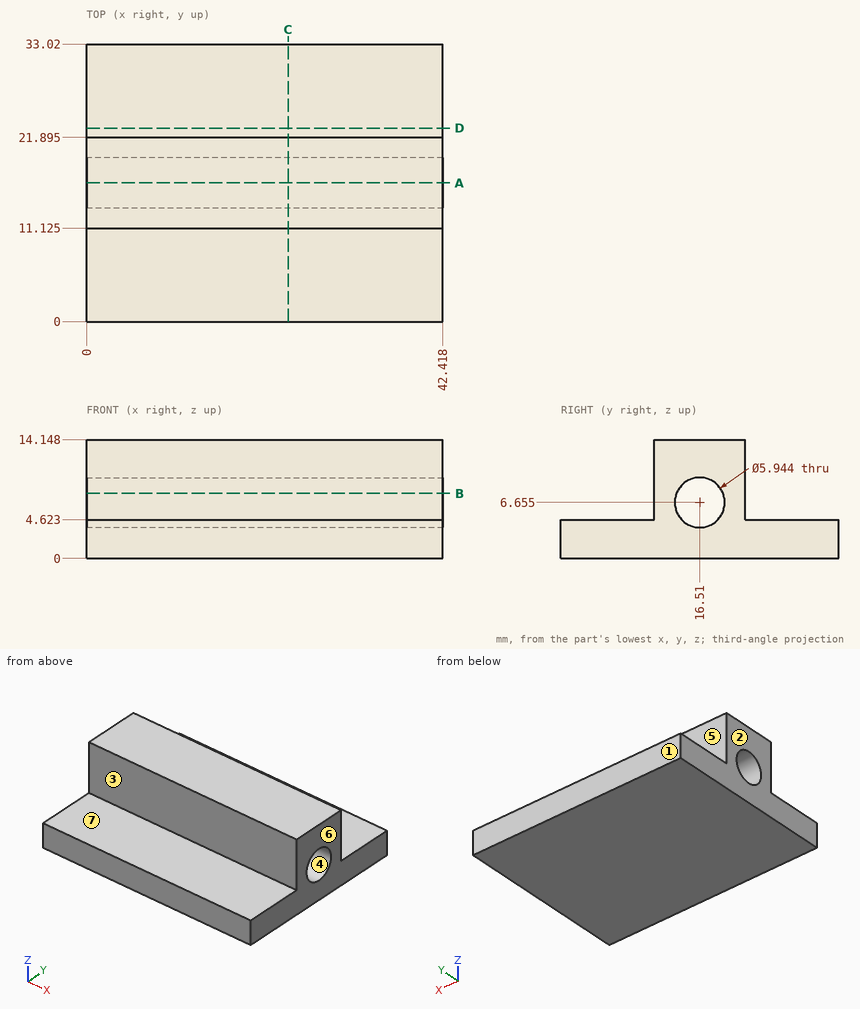
Verification items for this drawing (mm, ordinates from the low corner). A direction names the side the tool comes from. Coordinates: 2 decimals unless noted, no trailing zeros. Write each loop counter-clockwise with the first axis right and the second up, starting at its lowest first coordinate (ties: lowest second). Pieces come first, ordered by that corner, then holes. Notation, with made-up numbers: M 70,-5 L 126,-5 A29 ccw 126,17 Z; hole C 10,72 d6. An arc over 180 degrees is marked long. Answer as CSV lines item,"result".
Q1. Cross-section at D-D (y = 23). Record the boundary of the cut face in (x, z).
Check result:
outline,"M 0,0 L 42.42,0 L 42.42,4.62 L 0,4.62 Z"
Q2. Set-up check for the marked faces 5, 6 and 7: record each of +Z, -Z, +X, -X, +Y, -Y from which the full face is reachable in a straight line by a thin tool's end or side.
Check result:
face 5,"+Z, +X, -X, +Y"
face 6,"+Z, -Z, +X, +Y, -Y"
face 7,"+Z, +X, -X, -Y"
Q3. Material ranges on probe 1 along Y at (x, z) = (13.5, 11) (1 decimal); probe 2 along Z at (x, y) = (13, 16.51); probe 3 along Z at (x, y) = (11, 28.5), recorded low to high. Write a range as from..to.
Check result:
probe 1,"11.1..21.9"
probe 2,"0..3.68, 9.63..14.15"
probe 3,"0..4.62"
Q4. Cross-section at B-B (z = 7.75). Record the boundary of the cut face in (x, y) (1 decimal).
Check result:
outline,"M 0,11.1 L 42.4,11.1 L 42.4,13.7 L 0,13.7 Z; M 0,19.3 L 42.4,19.3 L 42.4,21.9 L 0,21.9 Z"
Q5. Cross-section at C-C (x = 24). Record the boundary of the cut face in (y, z) (1 decimal).
Check result:
outline,"M 0,0 L 33,0 L 33,4.6 L 21.9,4.6 L 21.9,14.1 L 11.1,14.1 L 11.1,4.6 L 0,4.6 Z; hole C 16.5,6.7 d5.9"
Q6. Go/stop test with flat-tipped pins: pin 1 (6 mm diameter, centred on x = 30.5, z = 10, fed in from +Y) (1 decimal); pin 2 (1 mm diameter, centred on x = 13.5, y = 16.5, fed in from -Z); pin 3 (3 mm diameter, centred on x = 14, z = 10.5, fed in from -Y) (1 decimal); pin 4 (3 mm diameter, centred on x = 27.5, y = 6.5, fed in from +Z). Record where each tip stops, or that it passes through.
Check result:
pin 1,"y = 21.9"
pin 2,"z = 0"
pin 3,"y = 11.1"
pin 4,"z = 4.62"
Q7. Cross-section at A-A (y = 16.51). Record the boundary of the cut face in (x, z), then the cut area to 3 significant figures.
Check result:
outline,"M 0,0 L 42.42,0 L 42.42,3.68 L 0,3.68 Z; M 0,9.63 L 42.42,9.63 L 42.42,14.15 L 0,14.15 Z"
area,"348 mm^2"
Q8. Mould release check, pull along Y, two halves, no side actions. Record for the marked faces 1, 2, 3 and 4: released by +Y, released by -Y, zero draft, split by the parting line, or undercut.
Check result:
face 1,"released by +Y"
face 2,"zero draft"
face 3,"released by -Y"
face 4,"undercut"
